Geometry: final body of the model. Coordinates: model frame, mm. Face numbers are marked on the shaded views. A direction names the side the tool comes from. Coordinates: 2 decimals unless noted, no trailing zeros. Loops run counter-clockwise (first coordinate to the right, second up) from the corner with the lowest first, then second, coordinate; pieces in that order, holes last. Notation, with made-up numbers: (-28.5, -7.5) - (-0.5, -7.5) arc R11 cw to (-0.5, 5.5) - close; hole circle Ø6 at (62, -36). An arc over 180 degrees is marked (long way). Answer in a Markdown table with one row per item.
from build123d import *

# Parameters (mm, degrees)
SKETCH1_R           = 6
SKETCH1_R_2         = 1.5
BOSS_EXTRUDE1_DEPTH = 1.5
FILLET1_R           = 7.5
FILLET2_R           = 1


with BuildPart() as part:
    # Sketch1 → Boss-Extrude1 (new, symmetric)
    with BuildSketch(Plane(origin=(0, 0, 0), x_dir=(0, 0, -1), z_dir=(1, 0, 0))):
        with BuildLine():
            Line((-7.5, 7.5), (7.5, 7.5))
            Line((7.5, 7.5), (7.5, 22.5))
            Line((7.5, 22.5), (-17.5, 22.5))
            ThreePointArc((-17.5, 22.5), (-24.571067812, 19.571067812), (-27.5, 12.5))
            Line((-27.5, 12.5), (-27.5, -9))
            Line((-27.5, -9), (-7.5, -9))
            Line((-7.5, -9), (-7.5, 7.5))
        make_face()
        with Locations((-17.5, 0)):
            Circle(SKETCH1_R, mode=Mode.SUBTRACT)
        with Locations((0, 15)):
            Circle(SKETCH1_R_2, mode=Mode.SUBTRACT)
    extrude(amount=BOSS_EXTRUDE1_DEPTH, both=True)

    # Fillet1
    fillet1_edges = [part.edges().sort_by_distance(p)[0] for p in [
        (0, -9, 27.5),
        (0, -9, 7.5),
        (0, 7.5, -7.5),
        (0, 22.5, -7.5),
    ]]
    fillet(fillet1_edges, radius=FILLET1_R - 0.0001)  # a hair under: the kernel refuses the full size

    # Fillet2
    fillet2_edges = [part.edges().sort_by_distance(p)[0] for p in [
        (0, 7.5, 7.5),
    ]]
    fillet(fillet2_edges, radius=FILLET2_R)


solid = part.part
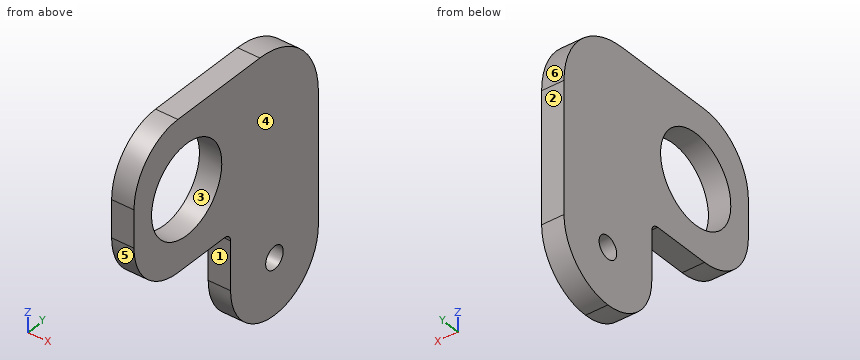
(1) Ray query, probe 1 along Y at (x, z) = (-0.7, 0); probe 2 along Y at (x, z) = (-0.4, 5); probe 3 along Z at (x, y) = (1.3, 2). Return the intervals inside material, ascending.
Verdict:
| item | result |
|---|---|
| probe 1 | y = 7.5 to 13.5, 16.5 to 22.5 |
| probe 2 | y = 7.5 to 22.5 |
| probe 3 | z = 7.5 to 11.84, 23.16 to 27.5 |
(2) Cut plane C-C on z = 4. Output: boundary loops of the cut face in (x, y).
Verdict:
| item | result |
|---|---|
| outline | (-1.5, 7.5) - (1.5, 7.5) - (1.5, 22.5) - (-1.5, 22.5) - close |
(3) Cut plane A-A on y = 0. Output: boundary loops of the cut face in (x, z).
Verdict:
| item | result |
|---|---|
| outline | (-1.5, 7.5) - (1.5, 7.5) - (1.5, 11.5) - (-1.5, 11.5) - close; (-1.5, 23.5) - (1.5, 23.5) - (1.5, 27.5) - (-1.5, 27.5) - close |
(4) Cut plane B-B on x = 0.75. State how many separate pieces and enclosed holes the cut face has, then the cut area to 3 significant figures.
Verdict:
| item | result |
|---|---|
| separate pieces | 1 |
| enclosed holes | 2 |
| area | 665 mm² |
(5) Pull-direction query (Y, two-part tool) for the marked faces 3, 4, 5 and 6; classes: pulls with the +Y half, pulls with the -Y half, needs draft (parallel to the pull), parting line crosses it, or undercut.
Verdict:
| item | result |
|---|---|
| face 3 | undercut |
| face 4 | needs draft |
| face 5 | pulls with the -Y half |
| face 6 | pulls with the +Y half |
(6) Cut plane D-D on y = -5.5. Output: boundary loops of the cut face in (x, z).
Verdict:
| item | result |
|---|---|
| outline | (-1.5, 8.66) - (1.5, 8.66) - (1.5, 15.1) - (-1.5, 15.1) - close; (-1.5, 19.9) - (1.5, 19.9) - (1.5, 26.34) - (-1.5, 26.34) - close |
(7) First-contact query: pin 1 Ø2.5 at (y, z) = (15, 0) entering from +X; pin 2 Ø1.5 at (x, y) = (-0.5, 1.5) entering from -Z; pin 3 Ø0.9 at (x, z) = (0, 4.5) entering from -Y. Flat tips, straight axial feed; report the tip coordinate or a pass-through.
Verdict:
| item | result |
|---|---|
| pin 1 | passes through |
| pin 2 | stops at z = 7.5 |
| pin 3 | stops at y = 7.5 |
(8) Access query for the marked faces 1 and 2. Directions: +Z, -Z, +X, -X, +Y, -Y. A direction counts if a zero-diameter tool reaches every point of the face in a straight line with its end or side. Return the directions, or none.
Verdict:
| item | result |
|---|---|
| face 1 | -Z, +X, -X, -Y |
| face 2 | +Z, -Z, +X, -X, +Y |
